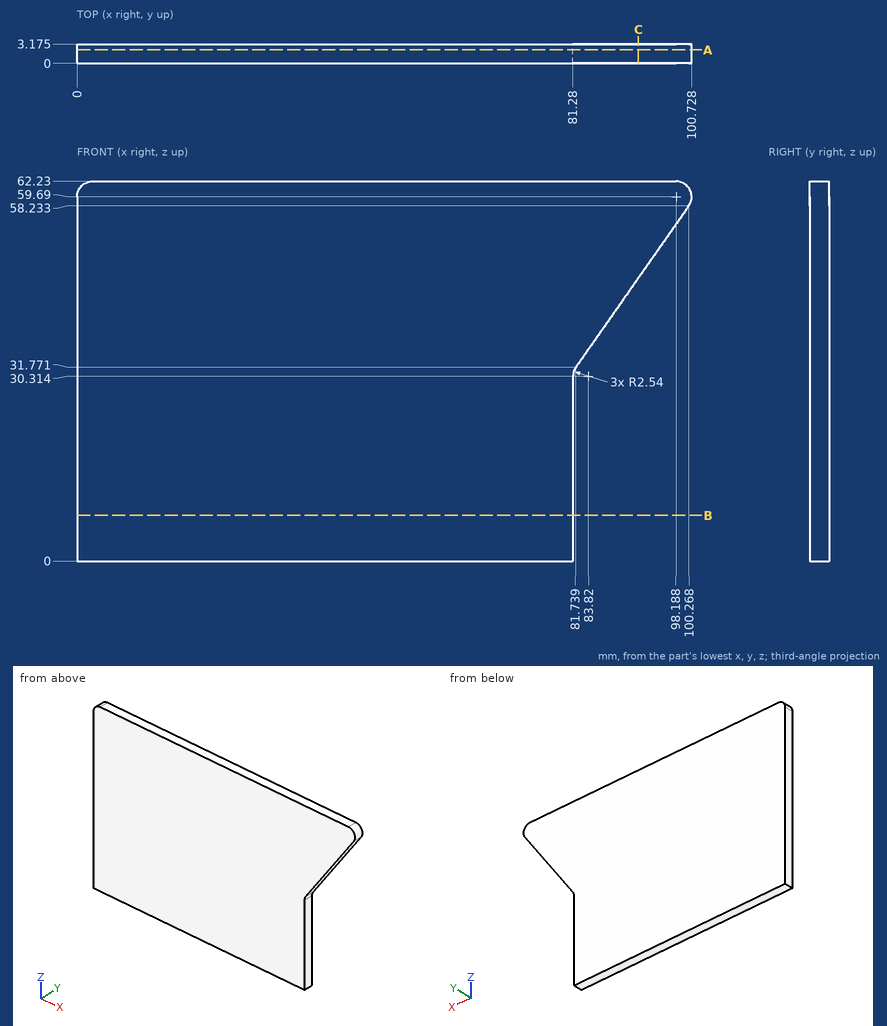
Geometry check sheet. Reference: drawing and pictorial views, mm from the part's lowest x, y, z. Round coordinates to 2 decimals unless told otherwise and drop trailing zeros. Write each loop counter-clockwise with the first axis right and the second up, starting at its lowest first coordinate (ties: lowest second). Pieces come first, ordered by that corner, then holes.
1. Section check C-C on x = 92. Enter the section's corners in (y, z) (1 decimal).
2. Section check A-A on y = 2.2. Enter the section's corners in (x, z).
3. Gauge pin test, flat end, axial feed: P1, Ø1.6, axis at y = 1.5, z = 13.5, coming from the +X side. Record the tip position at first contact, or that the pin passes through.
4. Scan lines: L1, parallel to X at y = 2.5, z = 4.5; L2, parallel to X at y = 1.85, z = 59. Record each from-to range of solid material in increasing order.
5. Section check B-B on z = 7.5. Enter the section's corners in (x, y) (1 decimal).
Answer:
1. outline: (0, 46.4) - (3.2, 46.4) - (3.2, 62.2) - (0, 62.2) - close
2. outline: (0, 0) - (81.28, 0) - (81.28, 30.31) arc R2.54 cw to (81.74, 31.77) - (100.27, 58.23) arc R2.54 ccw to (98.19, 62.23) - (2.54, 62.23) arc R2.54 ccw to (0, 59.69) - close
3. P1: stops at x = 81.28
4. L1: x = 0 to 81.28
4. L2: x = 0 to 100.63
5. outline: (0, 0) - (81.3, 0) - (81.3, 3.2) - (0, 3.2) - close
